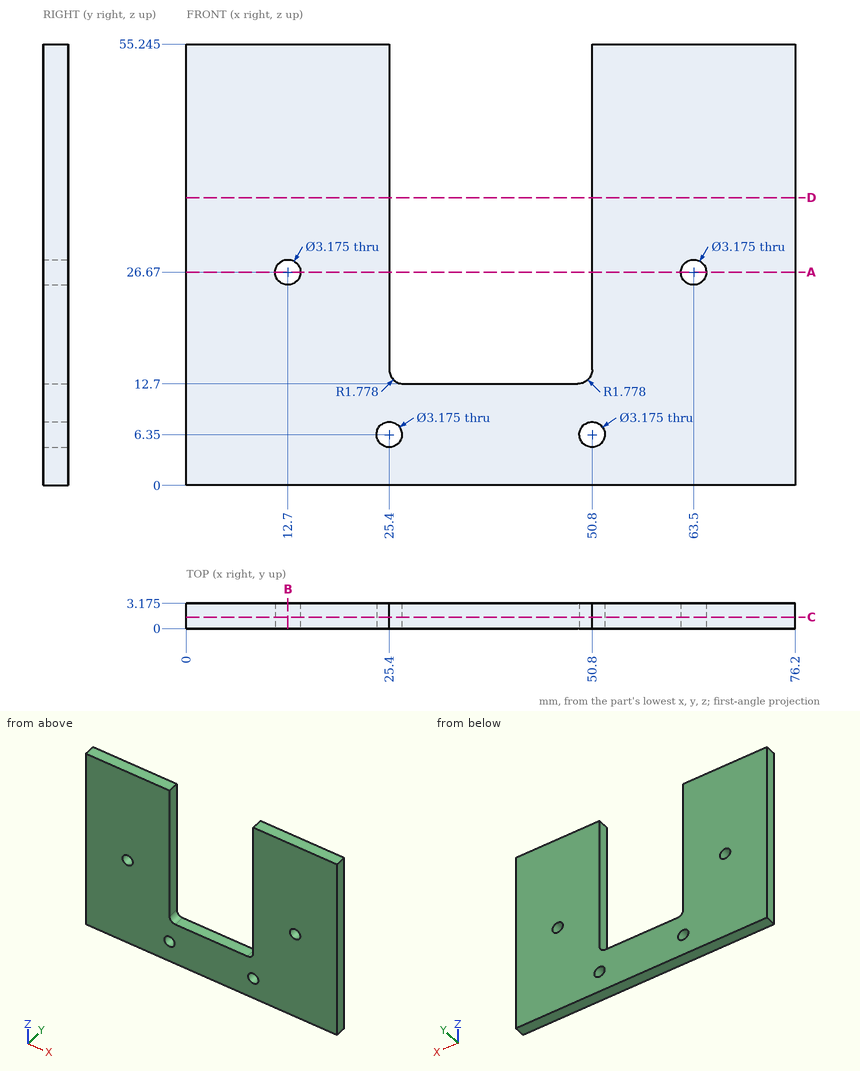
Job drawing, mm, ordinate dimensions from the low corner. One solid piece. Round coordinates to 2 decimals unless told otherwise and drop trailing zeros. Write each loop counter-clockwise with the first axis right and the second up, starting at its lowest first coordinate (ties: lowest second). Pieces come first, ordered by that corner, then holes. Notation, with made-up numbers: (42, -5.5) -> (95, -5.5) arc R19 cw to (95, 5.5) -> close; hole circle Ø6 at (-11.75, -33.5). An arc over 180 degrees is marked (long way). Answer as CSV lines item,"result".
1. Slice it at A-A, the plane z = 26.67. List the corners of the cut face in (x, y) (1 decimal).
Resolved:
outline,"(0, 0) -> (11.1, 0) -> (11.1, 3.2) -> (0, 3.2) -> close; (14.3, 0) -> (25.4, 0) -> (25.4, 3.2) -> (14.3, 3.2) -> close; (50.8, 0) -> (61.9, 0) -> (61.9, 3.2) -> (50.8, 3.2) -> close; (65.1, 0) -> (76.2, 0) -> (76.2, 3.2) -> (65.1, 3.2) -> close"
2. Slice it at B-B, the plane x = 12.7. List the corners of the cut face in (y, z) (1 decimal), plus the area to 3 significant figures.
Resolved:
outline,"(0, 0) -> (3.2, 0) -> (3.2, 25.1) -> (0, 25.1) -> close; (0, 28.3) -> (3.2, 28.3) -> (3.2, 55.2) -> (0, 55.2) -> close"
area,"165 mm²"
3. Drill centre lines: line 1 (X direction, y = 2.55, z = 26.67); line 2 (X direction, y = 1, z = 6.35); line 3 (X direction, y = 0.7, z = 25.5). Where is each one in solid material? Low to high.
Resolved:
line 1,"0 to 11.11, 14.29 to 25.4, 50.8 to 61.91, 65.09 to 76.2"
line 2,"0 to 23.81, 26.99 to 49.21, 52.39 to 76.2"
line 3,"0 to 11.63, 13.77 to 25.4, 50.8 to 62.43, 64.57 to 76.2"
4. Pin check, flat tips, straight feed: pin 1 Ø1 at (x, y) = (43, 1) entering from +Z; pin 2 Ø3 at (x, z) = (25.4, 6.35) entering from -Y. Stop position of each tip, or through.
Resolved:
pin 1,"z = 12.7"
pin 2,"through"
5. Slice it at C-C, the plane y = 1.45. State how many separate pieces and enclosed holes the cut face has, plus the area to 3 significant figures.
Resolved:
separate pieces,"1"
enclosed holes,"4"
area,"3,100 mm²"
6. Slice it at D-D, the plane z = 36. List the corners of the cut face in (x, y) (3 decimals), plus the area to 3 significant figures.
Resolved:
outline,"(0, 0) -> (25.4, 0) -> (25.4, 3.175) -> (0, 3.175) -> close; (50.8, 0) -> (76.2, 0) -> (76.2, 3.175) -> (50.8, 3.175) -> close"
area,"161 mm²"
